CAD build for the part. Positions are in the model's coordinates, mm. Face numbers are marked on the shaded views. A direction names the side the tool comes from. Give positions to 0.01 mm unless a question says otherwise; leave off trailing zeros. Order: outer loops, then holes, each group sorted by start corner. A loop starts at its lowest first (then second) coordinate and runs counter-clockwise, first axis right, second up.
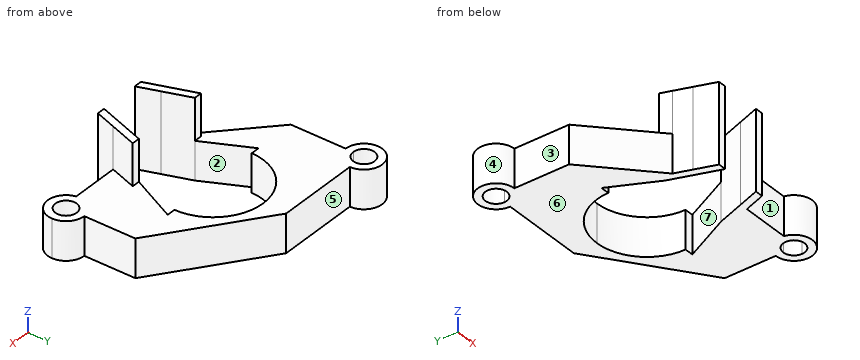
```python
from build123d import *

# Parameters (mm, degrees)
F1_DEPTH = 12
F2_DEPTH = 25


# Not quite as in the source:
# - ends of sketch curves that miss each other by under 0.0002 mm in the source are joined


with BuildPart() as f1:
    # F0 (on Top) → F1 (new body)
    with BuildSketch(Plane.XY):
        with BuildLine():
            ThreePointArc((-55.8174114415, 34.8348648238), (-58.1862191586, 40.5536725408), (-52.4674114416, 38.1848648238))
            Line((-52.4674114416, 38.1848648238), (-50.0674114416, 38.1848649627))
            ThreePointArc((-50.0674114416, 38.1848649627), (-59.8832754334, 42.2507288156), (-55.8174114415, 32.4348648238))
            Line((-55.8174114415, 32.4348648238), (-55.8174114415, 34.8348648238))
        make_face()
        with BuildLine():
            Line((-50.0674114416, 38.1848649627), (-52.4674114416, 38.1848649047))
            ThreePointArc((-52.4674114416, 38.1848649047), (-53.4486037246, 35.8160571069), (-55.8174114415, 34.8348648238))
            Line((-55.8174114415, 34.8348648238), (-55.8174114415, 32.4348648238))
            ThreePointArc((-55.8174114415, 32.4348648238), (-51.7515474497, 34.119000832), (-50.0674114416, 38.1848649627))
        make_face()
        with BuildLine():
            Line((-24.1338443596, 38.184865589), (-50.0674114416, 38.1848649627))
            ThreePointArc((-50.0674114416, 38.1848649627), (-51.7515474497, 34.119000832), (-55.8174114415, 32.4348648238))
            Line((-55.8174114415, 32.4348648238), (-55.8174114412, 15.1848640586))
            Line((-55.8174114412, 15.1848640586), (-42.6338443592, 15.1659585535))
            ThreePointArc((-42.6338443592, 15.1659585535), (-37.2153198113, 28.2474340054), (-24.1338443595, 33.6659585535))
            Line((-24.1338443595, 33.6659585535), (-24.1338443596, 38.184865589))
        make_face()
        with BuildLine():
            Line((-24.1338443595, 30.9159585535), (-24.1338443595, 33.6659585535))
            ThreePointArc((-24.1338443595, 33.6659585535), (-37.2153198113, 28.2474340054), (-42.6338443592, 15.1659585535))
            Line((-42.6338443592, 15.1659585535), (-39.8838443592, 15.1659585535))
            ThreePointArc((-39.8838443592, 15.1659585535), (-35.270776163, 26.3028903571), (-24.1338443595, 30.9159585535))
        make_face()
        with BuildLine():
            Line((7.5497227227, 15.1659585535), (-24.1338443596, 38.184865589))
            Line((-24.1338443596, 38.184865589), (-24.1338443595, 33.6659585535))
            ThreePointArc((-24.1338443595, 33.6659585535), (-11.0523689074, 28.2474340056), (-5.6338443592, 15.1659585535))
            Line((-5.6338443592, 15.1659585535), (7.5497227227, 15.1659585535))
        make_face()
        with BuildLine():
            ThreePointArc((-5.6338443592, 15.1659585535), (-11.0523689074, 28.2474340056), (-24.1338443595, 33.6659585535))
            Line((-24.1338443595, 33.6659585535), (-24.1338443595, 30.9159585535))
            ThreePointArc((-24.1338443595, 30.9159585535), (-12.9969125556, 26.3028903573), (-8.3838443592, 15.1659585535))
            Line((-8.3838443592, 15.1659585535), (-5.6338443592, 15.1659585535))
        make_face()
        with BuildLine():
            Line((7.549722723, -0.909568585), (7.5497227227, 15.1659585535))
            Line((7.5497227227, 15.1659585535), (-5.6338443592, 15.1659585535))
            Line((-5.6338443592, 15.1659585535), (-12.7387191109, 0.5919707473))
            Line((-12.7387191109, 0.5919707473), (-10.2387191109, 0.5919707473))
            Line((-10.2387191109, 0.5919707473), (-13.136122196, -7.8151351762))
            Line((-13.136122196, -7.8151351762), (1.9170354556, -7.8151351762))
            ThreePointArc((1.9170354556, -7.8151351762), (3.0939956275, -3.0251503303), (7.549722723, -0.909568585))
        make_face()
        Polygon((-42.6338443592, 15.1659585535), (-55.8174114412, 15.1848640586), (-36.8837256357, -2.690086035), (-38.0284454354, 0.643162408), (-35.5289696075, 0.5919707473), align=None)
        with BuildLine():
            ThreePointArc((13.2997227231, -6.659568585), (11.6155867149, -2.5937045931), (7.549722723, -0.909568585))
            ThreePointArc((7.549722723, -0.909568585), (3.0939956275, -3.0251503303), (1.9170354556, -7.8151351762))
            ThreePointArc((1.9170354556, -7.8151351762), (8.1304757738, -12.3801652229), (13.2997227231, -6.659568585))
        make_face()
        with BuildLine():
            ThreePointArc((10.8997227231, -6.659568585), (5.1809150061, -9.028376302), (7.549722723, -3.309568585))
            ThreePointArc((7.549722723, -3.309568585), (9.91853044, -4.290760868), (10.8997227231, -6.659568585))
        make_face(mode=Mode.SUBTRACT)
        Polygon((-38.0284454354, 0.643162408), (-36.8837256357, -2.690086035), (-35.1236572441, -7.8151351762), (-32.6315665225, -7.8151351762), (-35.5289696075, 0.5919707473), align=None)
        Polygon((-32.6315665225, -7.8151351762), (-35.1236572441, -7.8151351762), (-32.8838443592, -14.3371266833), (-30.3838443592, -14.3371266833), align=None)
        Polygon((-13.136122196, -7.8151351762), (-15.636122196, -7.8151351762), (-17.8838443592, -14.3371266833), (-15.3838443592, -14.3371266833), align=None)
        Polygon((-10.2387191109, 0.5919707473), (-12.7387191109, 0.5919707473), (-15.636122196, -7.8151351762), (-13.136122196, -7.8151351762), align=None)
    extrude(amount=F1_DEPTH)

    # F0 (on Top) → F2 (join)
    with BuildSketch(Plane.XY):
        Polygon((-38.0284454354, 0.643162408), (-36.8837256357, -2.690086035), (-35.1236572441, -7.8151351762), (-32.6315665225, -7.8151351762), (-35.5289696075, 0.5919707473), align=None)
        Polygon((-32.6315665225, -7.8151351762), (-35.1236572441, -7.8151351762), (-32.8838443592, -14.3371266833), (-30.3838443592, -14.3371266833), align=None)
        Polygon((-10.2387191109, 0.5919707473), (-12.7387191109, 0.5919707473), (-15.636122196, -7.8151351762), (-13.136122196, -7.8151351762), align=None)
        Polygon((-13.136122196, -7.8151351762), (-15.636122196, -7.8151351762), (-17.8838443592, -14.3371266833), (-15.3838443592, -14.3371266833), align=None)
    extrude(amount=F2_DEPTH)


solid = f1.part
```
Item 1: Slice it at D-D (x = -6.5). Give the cut face in (y, z).
Item 2: Slice it at A-A (z = 18.25). Give the cut face in (x, y).
Item 3: Two-plate mould, pull along X, no slides. Class the marked faces 1, 2, 3 and 4: released by +X, released by -X, zero draft, split by the parting line, or undercut.
Item 4: Slice it at C-C (y = 26.5). Give the cut face in (x, z).
Item 5: Wall check: L1, parallel to X at y = -6.5, z = 7.5; L2, parallel to Z at x = -49.5, y = 11; L3, parallel to X at y = 20, z = 10.75. Give the ranges that are in metal, low to high.
Item 6: Slice it at B-B (z = 10.5). Give the cut face in (x, y).
Item 7: Drop flat-ended pins along their axis: pin 1 Ø10 at (y, z) = (24, 4.5) entering from +X; pin 2 Ø9.5 at (x, z) = (-42, 7) entering from +Y; pin 3 Ø6 at (y, z) = (10.5, 7.5) entering from +X. Give the stop position or say it passes through.
Item 8: Tool access for the marked faces 5, 6 and 7: list every direction of +Z, -Z, +X, -X, +Y, -Y with a clear straight run to the whole face (end or side of a thin tool).
A:
1. outline: (-7.82, 0) - (13.39, 0) - (13.39, 12) - (-7.82, 12) - close; (15.17, 0) - (25.37, 0) - (25.37, 12) - (15.17, 12) - close
2. outline: (-38.03, 0.64) - (-32.88, -14.34) - (-30.38, -14.34) - (-35.53, 0.59) - close; (-17.88, -14.34) - (-15.38, -14.34) - (-10.24, 0.59) - (-12.74, 0.59) - close
3. face 1: undercut
3. face 2: undercut
3. face 3: released by -X
3. face 4: split by the parting line
4. outline: (-55.82, 0) - (-35.07, 0) - (-35.07, 12) - (-55.82, 12) - close; (-13.2, 0) - (-8.05, 0) - (-8.05, 12) - (-13.2, 12) - close
5. L1: x = -35.58 to -33.08, -15.18 to 4.2, 10.9 to 13.3
5. L2: z = 0 to 12
5. L3: x = -55.82 to -39.12, -9.14 to 0.9
6. outline: (-55.82, 15.18) - (-36.88, -2.69) - (-32.88, -14.34) - (-30.38, -14.34) - (-35.53, 0.59) - (-42.63, 15.17) - (-39.88, 15.17) arc R15.75 cw to (-8.38, 15.17) - (-5.63, 15.17) - (-12.74, 0.59) - (-17.88, -14.34) - (-15.38, -14.34) - (-13.14, -7.82) - (1.92, -7.82) arc R5.75 ccw (long way) to (7.55, -0.91) - (7.55, 15.17) - (-24.13, 38.18) - (-50.07, 38.18) arc R5.75 ccw (long way) to (-55.82, 32.43) - close; hole circle Ø6.7 at (-55.82, 38.18); hole circle Ø6.7 at (7.55, -6.66)
7. pin 1: stops at x = 2.27
7. pin 2: stops at y = 38.18
7. pin 3: stops at x = 7.55
8. face 5: +Z, -Z, +X, +Y
8. face 6: -Z, +X, -X, +Y, -Y
8. face 7: +Z, -Z
